from build123d import *

# Parameters (mm, degrees)
BOSS_EXTRUDE1_DEPTH = 60
SKETCH3_R           = 7.5
CUT_EXTRUDE1_DEPTH  = 49


with BuildPart() as part:
    # Sketch1 → Boss-Extrude1 (new body)
    with BuildSketch(Plane(origin=(0, 0, 0), x_dir=(0, 0, -1), z_dir=(1, 0, 0))):
        Polygon((-5, 7.5), (0, 7.5), (0, 10), (38, 10), (38, 0), (43, 0), (43, 15), (-5, 15), align=None)
        Polygon((43, 0), (38, 0), (38, -10), (0, -10), (0, -7.5), (-5, -7.5), (-5, -15), (43, -15), align=None)
    extrude(amount=BOSS_EXTRUDE1_DEPTH)

    # Sketch3 → Cut-Extrude1 (cut, through all)
    with BuildSketch(Plane(origin=(0, 0, -43), x_dir=(-1, 0, 0), z_dir=(0, 0, -1))):
        with Locations((-48.743612904, 0)):
            Circle(SKETCH3_R)
    extrude(amount=-CUT_EXTRUDE1_DEPTH, mode=Mode.SUBTRACT)


solid = part.part
Can you work these out from the model? Positions are in its coordinate system, mm. A direction names the side the tool comes from. Give positions to 0.01 mm unless a question says otherwise; leave off trailing zeros. Loops run counter-clockwise (first coordinate to the right, second up) from the corner with the lowest first, then second, coordinate; pieces in that order, holes last. Notation, with made-up numbers: (-6, -14.5) - (4, -14.5) arc R21 ccw to (4, 1.5) - close; hole circle Ø2 at (61, 89). An arc over 180 degrees is marked (long way). Return JSON: item names as keys, results as strings.
1. I want a section at D-D on x = 42.5. Please give me the cut outline in (y, z), and give its area (3 significant figures).
Output values:
{"outline": "(-15, -43) - (-4.16, -43) - (-4.16, -38) - (-10, -38) - (-10, 0) - (-7.5, 0) - (-7.5, 5) - (-15, 5) - close; (4.16, -43) - (15, -43) - (15, 5) - (7.5, 5) - (7.5, 0) - (10, 0) - (10, -38) - (4.16, -38) - close", "area": "563 mm²"}
2. I want a section at A-A on z = -32. Please give me the cut outline in (x, y).
Output values:
{"outline": "(0, -15) - (60, -15) - (60, -10) - (0, -10) - close; (0, 10) - (60, 10) - (60, 15) - (0, 15) - close"}
3. For faces 4 (the face through (30, 7.5, 3)), 5 (the face through (30, -15, -19)), 6 (the face through (30, -9, 0)), which set-ups out of +Z, -Z, +X, -X, +Y, -Y let a thin tool reach every point of the face, with its end or its side?
Output values:
{"face 4": "+Z, +X, -X", "face 5": "+Z, -Z, +X, -X, -Y", "face 6": "+X, -X"}
4. I'm going to push flat-ended pins straight in: pin 1 Ø12 at (x, y) = (48.74, 0) entering from -Z; pin 2 Ø1.5 at (x, y) = (42.5, -3.5) entering from +Z. Where does each tip first touch, or does it pass through?
Output values:
{"pin 1": "passes through", "pin 2": "stops at z = -38"}
5. If I drill on line 1 (Y direction, x = 23, z = -20); line 2 (Z direction, x = 14, y = 9.5); line 3 (Z direction, x = 30.5, y = -4.5), over which ranges is the centre line in solid material (lowest first)?
Output values:
{"line 1": "y = -15 to -10, 10 to 15", "line 2": "z = -43 to -38, 0 to 5", "line 3": "z = -43 to -38"}
6. I want a section at B-B on y = 0. Please give me the cut outline in (x, z).
Output values:
{"outline": "(0, -43) - (41.24, -43) - (41.24, -38) - (0, -38) - close; (56.24, -43) - (60, -43) - (60, -38) - (56.24, -38) - close"}
7. We'd pull the mould along Z, two halves only. Please class faces 1 (the face through (30, -11, 5)), 2 (the face through (30, 10, -19)), 3 (the face through (60, 10.2, -24)): +Z half, -Z half, draft (parallel to the pull), parting line (faces both ways), or undercut.
Output values:
{"face 1": "+Z half", "face 2": "undercut", "face 3": "draft"}
8. I want a section at C-C on x = 20. Please give me the cut outline in (y, z).
Output values:
{"outline": "(-15, -43) - (15, -43) - (15, 5) - (7.5, 5) - (7.5, 0) - (10, 0) - (10, -38) - (-10, -38) - (-10, 0) - (-7.5, 0) - (-7.5, 5) - (-15, 5) - close"}
